Check sheet for the drawn part. Datum: minimum x, y, z corner. Units: mm. A direction names the side the tool comes from. Give positions to 0.01 mm unless a question says otherwise; leave off trailing zeros. Write each loop counter-clockwise with the first axis right and the second up, starting at its lowest first coordinate (ties: lowest second). Pieces come first, ordered by that corner, then holes. Notation, with made-up numbers: (-35, -1.5) -> (-15, -1.5) arc R26 ccw to (-15, 17.5) -> close; hole circle Ø10 at (-12, 44.25). An arc over 180 degrees is marked (long way). Answer as CSV lines item,"result". Start each with the question number.
1) Sectioned sample at A-A on y = 3.25. Record the cut outline in (x, z).
2) Tool access check on the marked faces 1 and 2. Record the directions out of +Z, -Z, +X, -X, +Y, -Y that give a thin tool (end or side, any length) a straight path to the whole face; none if there is none.
3) Sectioned sample at C-C on z = 11.75. Record the cut outline in (x, y).
4) Sectioned sample at D-D on y = 0.45. Record the cut outline in (x, z), and give its area (3 significant figures).
5) Material ranges on L1, parallel to Z at x = 5, y = 1.7; L2, parallel to Y at x = 1.75, z = 5.5; L3, parallel to X at y = 1, z = 3, recorded low to high.
6) Sectioned sample at B-B on x = 4.32. Record the cut outline in (y, z), and give its area (3 significant figures).
7) Gauge pin test, flat end, axial feed: pin 1 Ø2 at (y, z) = (4, 11) entering from +X. Record the tip position at first contact, or that the pin passes through.
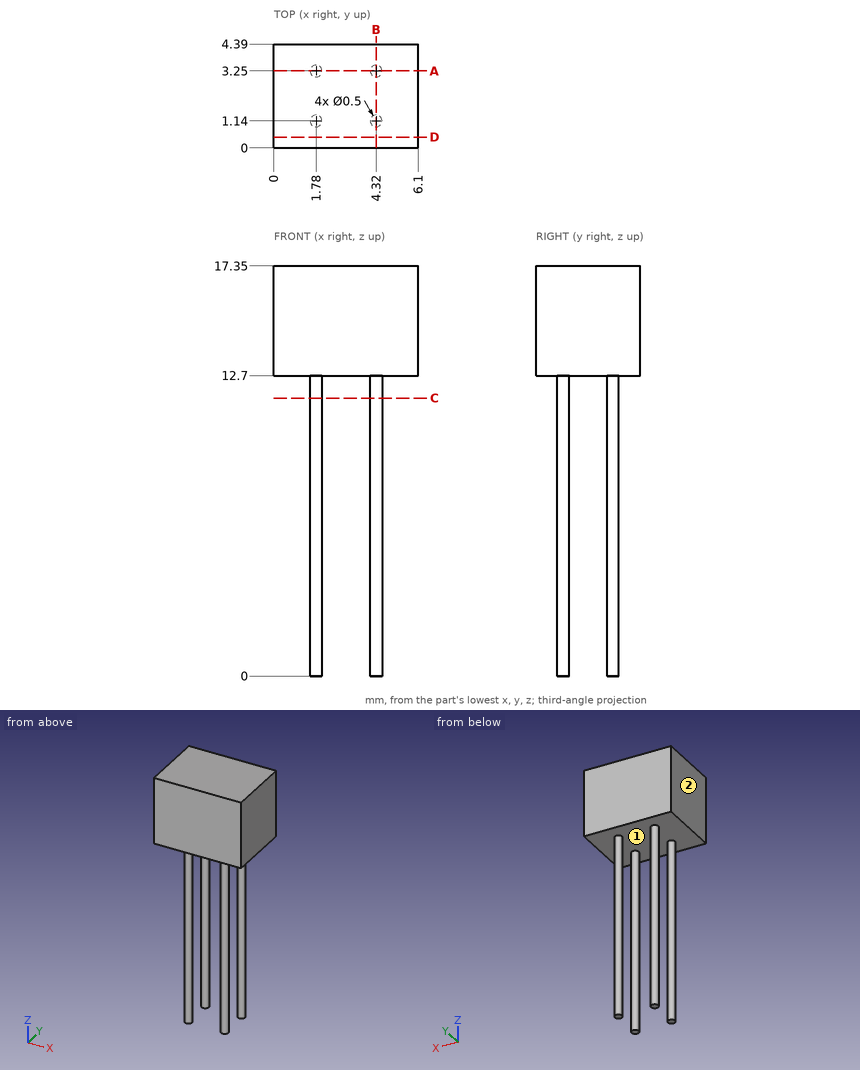
Ans:
1,outline,"(0, 12.7) -> (1.53, 12.7) -> (1.53, 0) -> (2.03, 0) -> (2.03, 12.7) -> (4.07, 12.7) -> (4.07, 0) -> (4.57, 0) -> (4.57, 12.7) -> (6.1, 12.7) -> (6.1, 17.35) -> (0, 17.35) -> close"
2,face 1,"-Z"
2,face 2,"+Z, -Z, -X, +Y, -Y"
3,outline,"circle Ø0.5 at (1.78, 1.14); circle Ø0.5 at (1.78, 3.25); circle Ø0.5 at (4.32, 1.14); circle Ø0.5 at (4.32, 3.25)"
4,outline,"(0, 12.7) -> (6.1, 12.7) -> (6.1, 17.35) -> (0, 17.35) -> close"
4,area,"28.4 mm²"
5,L1,"z = 12.7 to 17.35"
5,L2,"y = 0.89 to 1.39, 3 to 3.5"
5,L3,"x = 1.57 to 1.99, 4.11 to 4.53"
6,outline,"(0, 12.7) -> (0.89, 12.7) -> (0.89, 0) -> (1.39, 0) -> (1.39, 12.7) -> (3, 12.7) -> (3, 0) -> (3.5, 0) -> (3.5, 12.7) -> (4.39, 12.7) -> (4.39, 17.35) -> (0, 17.35) -> close"
6,area,"33.1 mm²"
7,pin 1,"stops at x = 4.57"
